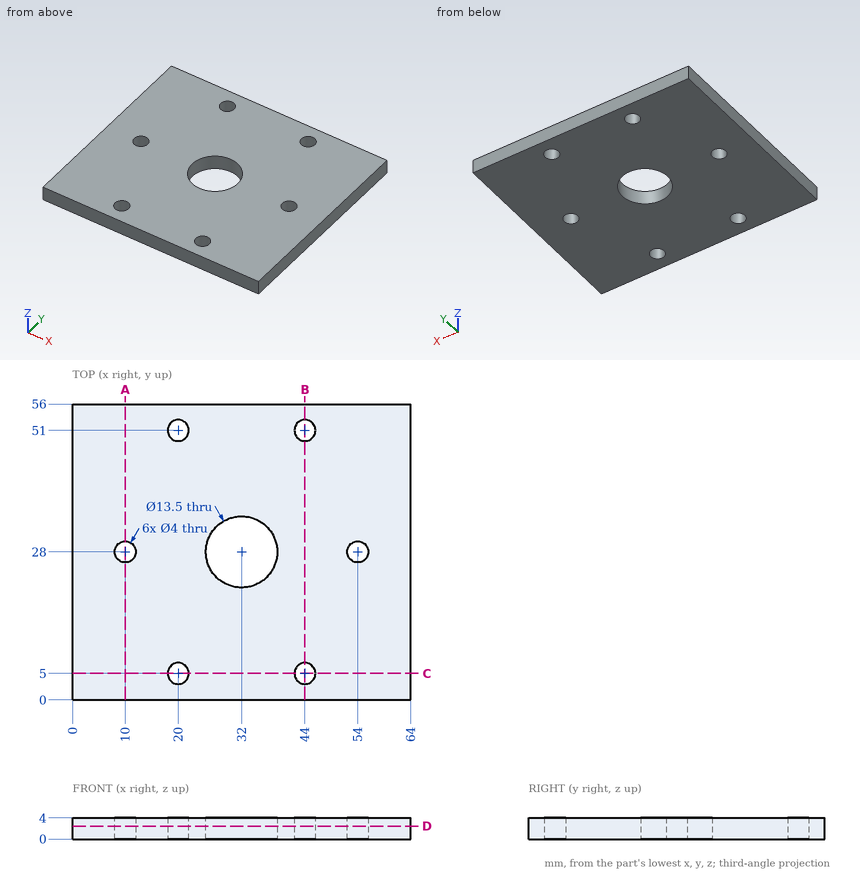
The drawing under review shows one solid part. Ordinate dimensions are in mm from its lowest x, y, z. Round coordinates to 2 decimals unless told otherwise and drop trailing zeros. Write each loop counter-clockwise with the first axis right and the second up, starting at its lowest first coordinate (ties: lowest second). Pieces come first, ordered by that corner, then holes.
(1) We need section C-C on y = 5. Give the boundary of the cut face in (x, z), and give its area (3 significant figures).
(2) Insertion check: pin 1 (2 mm diameter, centred on x = 12.5, y = 9.5, fed in from -Z). The pin has a flat end and moves straight along its axis. Give the tip position at first contact, or say it passes through.
(3) We need section B-B on x = 44. Give the boundary of the cut face in (y, z).
(4) We need section D-D on z = 2.45. Give the boundary of the cut face in (x, y), and give its area (3 significant figures).
(5) Wall thickness on L1, parallel to Y at x = 20, z = 2.6; L2, parallel to Y at x = 32, z = 2.6; L3, parallel to X at y = 29, z = 1.4: over which ranges is each line inside the solid? List them lowest first.
(6) We need section A-A on x = 10. Give the boundary of the cut face in (y, z), and give its area (3 significant figures).
Findings below:
1. outline: (0, 0) - (18, 0) - (18, 4) - (0, 4) - close; (22, 0) - (42, 0) - (42, 4) - (22, 4) - close; (46, 0) - (64, 0) - (64, 4) - (46, 4) - close
1. area: 224 mm2
2. pin 1: stops at z = 0
3. outline: (0, 0) - (3, 0) - (3, 4) - (0, 4) - close; (7, 0) - (49, 0) - (49, 4) - (7, 4) - close; (53, 0) - (56, 0) - (56, 4) - (53, 4) - close
4. outline: (0, 0) - (64, 0) - (64, 56) - (0, 56) - close; hole circle Ø4 at (10, 28); hole circle Ø4 at (20, 5); hole circle Ø4 at (20, 51); hole circle Ø13.5 at (32, 28); hole circle Ø4 at (44, 5); hole circle Ø4 at (44, 51); hole circle Ø4 at (54, 28)
4. area: 3,370 mm2
5. L1: y = 0 to 3, 7 to 49, 53 to 56
5. L2: y = 0 to 21.25, 34.75 to 56
5. L3: x = 0 to 8.27, 11.73 to 25.32, 38.68 to 52.27, 55.73 to 64
6. outline: (0, 0) - (26, 0) - (26, 4) - (0, 4) - close; (30, 0) - (56, 0) - (56, 4) - (30, 4) - close
6. area: 208 mm2
